Input: part model. Units: mm. Frame: model coordinates. Face numbers are marked on the shaded views. A direction names the side the tool comes from. Round coordinates to 2 decimals unless told otherwise and drop trailing zeros. Write each loop counter-clockwise with the first axis right and the second up, starting at its lowest first coordinate (ties: lowest second). Pieces come first, ordered by that corner, then holes. Notation, with made-up numbers: (27.5, 32.5) - (74.5, 32.5) arc R29 cw to (74.5, 63.5) - close; hole circle Ø4 at (51.25, 25.25). An arc over 180 degrees is marked (long way). Use one line per item in the form item = value.
```python
from build123d import *

# Parameters (mm, degrees)
F0_W     = 25
F0_H     = 8
F1_DEPTH = 5
F2_SIZE  = 2
F3_SIZE  = 2
F4_W     = 2
F4_H     = 4
F5_DEPTH = 25


with BuildPart() as f1:
    # F0 (on Front) → F1 (new body, symmetric)
    with BuildSketch(Plane.XZ):
        with Locations((0, 30)):
            Rectangle(F0_W, F0_H)
    extrude(amount=F1_DEPTH, both=True)

    # F2
    f2_edges = [f1.edges().sort_by_distance(p)[0] for p in [
        (12.5, 0, 26),
        (-12.5, 0, 26),
    ]]
    chamfer(f2_edges, length=F2_SIZE)

    # F3
    f3_edges = [f1.edges().sort_by_distance(p)[0] for p in [
        (0, -5, 26),
        (0, 5, 26),
    ]]
    chamfer(f3_edges, length=F3_SIZE)

    # F4 (on face) → F5 (cut)
    with BuildSketch(Plane(origin=(-12.5, 0, 0), x_dir=(0, -1, 0), z_dir=(-1, 0, 0))):
        with Locations((4, 32)):
            Rectangle(F4_W, F4_H)
        with Locations((-4, 32)):
            Rectangle(F4_W, F4_H)
        Polygon((-0.38, 33), (0, 33), (0.38, 33), (0.38, 34), (-0.38, 34), align=None)
    extrude(amount=-F5_DEPTH, mode=Mode.SUBTRACT)


solid = f1.part
```
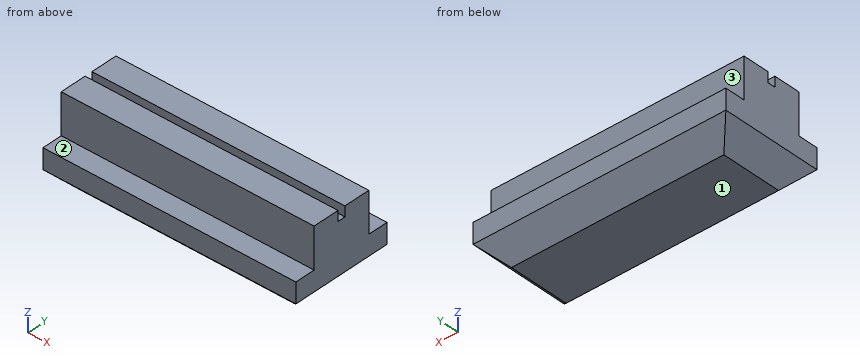
(1) Access query for the marked faces 1, 2 and 3. Directions: +Z, -Z, +X, -X, +Y, -Y. A direction counts if a zero-diameter tool reaches every point of the face in a straight line with its end or side. Return the directions, or none.
Derived:
face_1 = -Z, +X, -X, +Y, -Y
face_2 = +Z, +X, -X, -Y
face_3 = +Z, +X, -X, +Y
(2) Cut plane C-C on z = 27.5. Output: boundary loops of the cut face in (x, y).
Derived:
outline = (-12, -4.5) - (12, -4.5) - (12, 4.5) - (-12, 4.5) - close
(3) First-contact query: pin 1 Ø1.6 at (x, y) = (-3.5, -4) entering from +Z; pin 2 Ø1.1 at (x, z) = (4.5, 33.5) entering from -Y; pin 3 Ø0.5 at (x, z) = (-1.5, 33.5) entering from +Y. Flat tips, straight axial feed; report the tip coordinate or a pass-through.
Derived:
pin_1 = 30
pin_2 = -3
pin_3 = 3
(4) Material intervals for L1, parallel to Y at x = -9.25, z = 31; L2, parallel to Z at x = -5, y = 0.25; L3, parallel to Z at x = -10.25, y = 3.25, sorted ascending.
Derived:
L1 = -3 to 3
L2 = 26 to 33
L3 = 26.25 to 30
(5) Cut plane B-B on y = 0. Output: boundary loops of the cut face in (x, z), then the cut area to 3 significant figures.
Derived:
outline = (-12.5, 28) - (-10.5, 26) - (10.5, 26) - (12.5, 28) - (12.5, 33) - (-12.5, 33) - close
area = 171 mm^2
(6) Cut plane D-D on y = -3.5. Output: boundary loops of the cut face in (x, z).
Derived:
outline = (-12.5, 28) - (-11, 26.5) - (11, 26.5) - (12.5, 28) - (12.5, 30) - (-12.5, 30) - close
(7) Cut plane A-A on x = -9. Output: boundary loops of the cut face in (y, z).
Derived:
outline = (-5, 28) - (-3, 26) - (3, 26) - (5, 28) - (5, 30) - (3, 30) - (3, 34) - (0.38, 34) - (0.38, 33) - (-0.38, 33) - (-0.38, 34) - (-3, 34) - (-3, 30) - (-5, 30) - close
